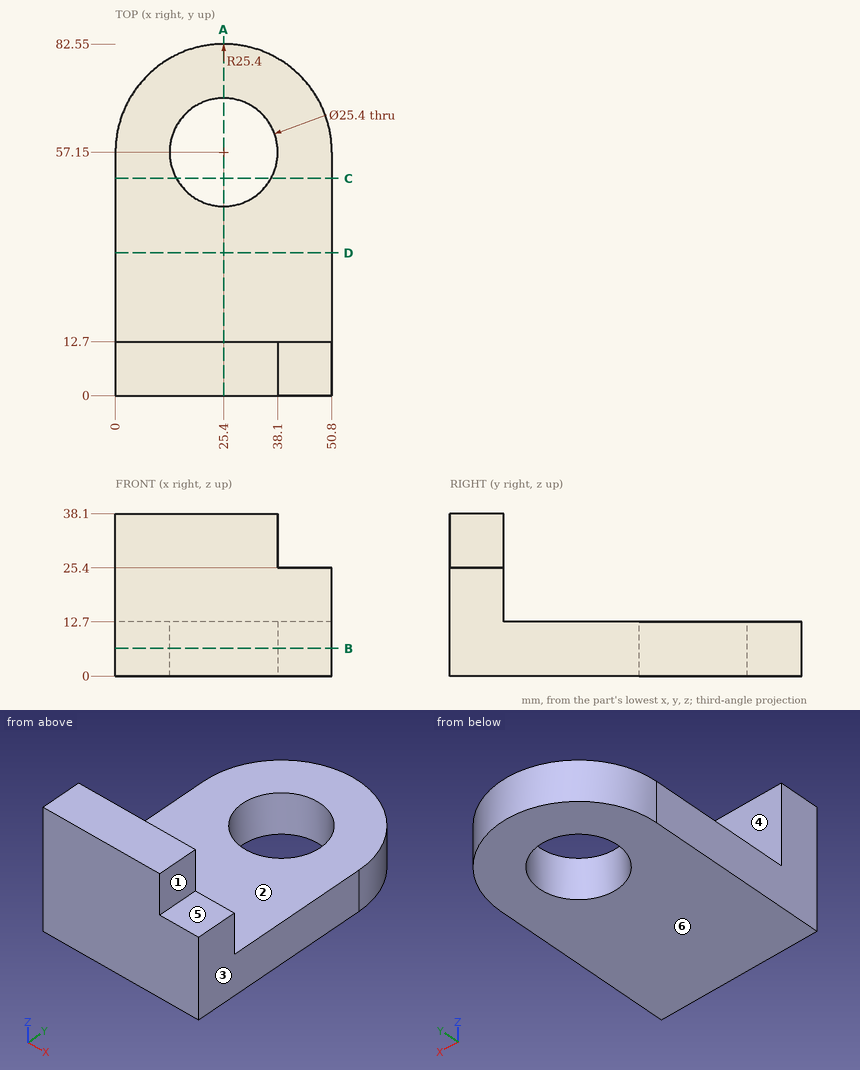
Answer from the drawing. Dimensions are ordinates in mm from the lowest x, y and z of the part. A direction names the side the tool comes from. Round coordinates to 2 decimals unless told otherwise and drop trailing zeros. Write each loop counter-clockwise with the first axis right and the second up, starting at its lowest first coordinate (ties: lowest second). Pieces come first, ordered by that corner, then holes. Notation, with made-up numbers: (-17, 12) -> (21, 12) arc R36 cw to (21, 48) -> close; hole circle Ø2 at (-2.5, -26). An arc over 180 degrees is marked (long way). Answer in a Markdown table with one row per item. Add a question column.
1) Find section B-B, the plane z = 6.5. Determine the outline of the cut face in (x, y), and give its area (3 significant figures).
2) Find section D-D, the plane y = 33.5. Determine the outline of the cut face in (x, z).
3) Which of the six approach directions +Z, -Z, +X, -X, +Y, -Y give full straight-line access (tool end or side, diameter ignored) to the marked faces 1, 2 and 3?
4) Consider line 1 (Y direction, x = 25.4, z = 7.75); line 2 (Z direction, x = 48, y = 41). Determine where each line is inside the solid, lowest interval first.
5) Find section A-A, the plane x = 25.4. Determine the outline of the cut face in (y, z).
6) Given P1, Ø10, axis at x = 45.5, y = 10, coming from the +Z side; P2, Ø6.5, axis at y = 5, z = 32.5, coming from the +X side; P3, Ø1.5, axis at x = 31, y = 36, coming from the +Z side, each flat-ended and moving along its own axis, determine where each tip first touches the part or whether it passes through.
7) Determine the mould class of the marked faces 4, 5 and 6 for opening direction Z: pulls with the +Z half, pulls with the -Z half, needs draft (parallel to the pull), parting line crosses it, or undercut.
8) Find section C-C, the plane y = 51. Determine the outline of the cut face in (x, z), and give its area (3 significant figures).
Findings below:
| question | item | result |
|---|---|---|
| 1 | outline | (0, 0) -> (50.8, 0) -> (50.8, 57.15) arc R25.4 ccw to (0, 57.15) -> close; hole circle Ø25.4 at (25.4, 57.15) |
| 1 | area | 3,410 mm² |
| 2 | outline | (0, 0) -> (50.8, 0) -> (50.8, 12.7) -> (0, 12.7) -> close |
| 3 | face 1 | +Z, +X, +Y, -Y |
| 3 | face 2 | +Z, +X, -X, +Y |
| 3 | face 3 | +Z, -Z, +X, +Y, -Y |
| 4 | line 1 | 0 to 44.45, 69.85 to 82.55 |
| 4 | line 2 | 0 to 12.7 |
| 5 | outline | (0, 0) -> (44.45, 0) -> (44.45, 12.7) -> (12.7, 12.7) -> (12.7, 38.1) -> (0, 38.1) -> close; (69.85, 0) -> (82.55, 0) -> (82.55, 12.7) -> (69.85, 12.7) -> close |
| 6 | P1 | z = 25.4 |
| 6 | P2 | x = 38.1 |
| 6 | P3 | z = 12.7 |
| 7 | face 4 | needs draft |
| 7 | face 5 | pulls with the +Z half |
| 7 | face 6 | pulls with the -Z half |
| 8 | outline | (0, 0) -> (14.29, 0) -> (14.29, 12.7) -> (0, 12.7) -> close; (36.51, 0) -> (50.8, 0) -> (50.8, 12.7) -> (36.51, 12.7) -> close |
| 8 | area | 363 mm² |
